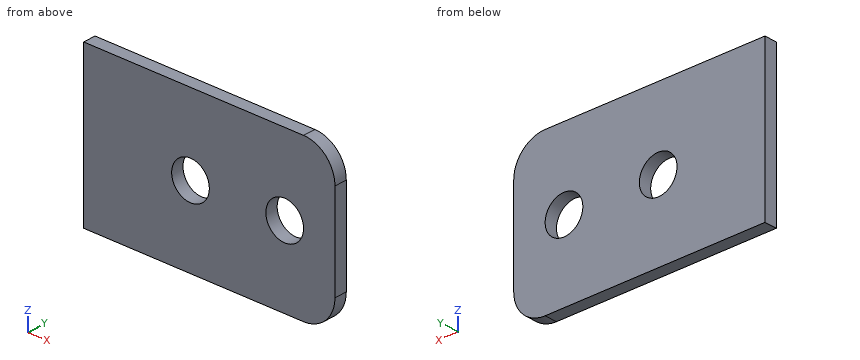
```python
from build123d import *

# Parameters (mm, degrees)
CYLINDER001_R     = 3
CYLINDER001_DEPTH = 10
CYLINDER002_R     = 3
CYLINDER002_DEPTH = 10
BOX_W             = 40
BOX_H             = 2
BOX_DEPTH         = 25
FILLET_R          = 5


with BuildPart() as cylinder001:
    # Cylinder001 → Cylinder001 (new body)
    with BuildSketch(Plane(origin=(32, -5, 12.5), x_dir=(1, 0, 0), z_dir=(0, 1, 0))):
        Circle(CYLINDER001_R)
    extrude(amount=CYLINDER001_DEPTH)


with BuildPart() as compound:
    # Cylinder002 → Cylinder002 (new body)
    with BuildSketch(Plane(origin=(17, -5, 12.5), x_dir=(1, 0, 0), z_dir=(0, 1, 0))):
        Circle(CYLINDER002_R)
    extrude(amount=CYLINDER002_DEPTH)

    # Compound: union Cylinder001
    add(cylinder001.part)


with BuildPart() as cut:
    # Box → Box (new body)
    with BuildSketch(Plane(origin=(0, -1, 0), x_dir=(1, 0, 0), z_dir=(0, 0, 1))):
        with Locations((20, 1)):
            Rectangle(BOX_W, BOX_H)
    extrude(amount=BOX_DEPTH)

    # Fillet
    fillet_edges = [cut.edges().sort_by_distance(p)[0] for p in [
        (40, 0, 25),
        (40, 0, 0),
    ]]
    fillet(fillet_edges, radius=FILLET_R)

    # Cut: cut Compound
    add(compound.part, mode=Mode.SUBTRACT)


with BuildPart() as cut_1:
    # Cut placement: moved
    add(cut.part.moved(Location((10, 0, 3))))


solid = cut_1.part
```
For this review, take the finished solid that the model builds, in its own axes (mm). Give positions to 0.01 mm unless a question says otherwise; leave off trailing zeros. Write each loop counter-clockwise with the first axis right and the second up, starting at its lowest first coordinate (ties: lowest second). Pieces come first, ordered by that corner, then holes. Notation, with made-up numbers: M 73,13.25 L 126,13.25 A12 ccw 126,19.25 Z; hole C 80,18 d8. An arc over 180 degrees is marked long. Answer as CSV lines item,"result".
1. Consider section A-A, the plane x = 42. Write out the cut boundary in (y, z).
Findings:
outline,"M -1,3 L 1,3 L 1,12.5 L -1,12.5 Z; M -1,18.5 L 1,18.5 L 1,28 L -1,28 Z"
2. Consider section D-D, the plane z = 4.5. Write out the cut boundary in (x, y).
Findings:
outline,"M 10,-1 L 48.57,-1 L 48.57,1 L 10,1 Z"
3. Consider section C-C, the plane z = 17. Write out the cut boundary in (x, y), then the cut area to 3 significant figures.
Findings:
outline,"M 10,-1 L 24.4,-1 L 24.4,1 L 10,1 Z; M 29.6,-1 L 39.4,-1 L 39.4,1 L 29.6,1 Z; M 44.6,-1 L 50,-1 L 50,1 L 44.6,1 Z"
area,"59.2 mm2"
4. Consider section B-B, the plane y = 0.05. Write out the cut boundary in (x, z).
Findings:
outline,"M 10,3 L 45,3 A5 ccw 50,8 L 50,23 A5 ccw 45,28 L 10,28 Z; hole C 27,15.5 d6; hole C 42,15.5 d6"
5. Wall thickness on line 1 (Z direction, x = 27, y = -0.4); line 2 (X direction, y = 0.6, z = 15.75); line 3 (X direction, y = 0.55, z = 13.25): over which ranges is each line inside the solid? List them lowest first.
Findings:
line 1,"z = 3 to 12.5, 18.5 to 28"
line 2,"x = 10 to 24.01, 29.99 to 39.01, 44.99 to 50"
line 3,"x = 10 to 25.02, 28.98 to 40.02, 43.98 to 50"
